from build123d import *

# Parameters (mm, degrees)
F0_R     = 3
F1_DEPTH = 18
F2_R     = 2.1
F3_DEPTH = 10
F4_R     = 1.4
F5_DEPTH = 18.001
F6_SIZE  = 0.5
F7_SIZE  = 0.5


with BuildPart() as f1:
    # F0 (on Front) → F1 (new body)
    with BuildSketch(Plane.XZ):
        Circle(F0_R)
    extrude(amount=-F1_DEPTH)

    # F2 (on face) → F3 (cut)
    with BuildSketch(Plane.XZ):
        Circle(F2_R)
    extrude(amount=-F3_DEPTH, mode=Mode.SUBTRACT)

    # F4 (on Front) → F5 (cut, through all)
    with BuildSketch(Plane.XZ):
        Circle(F4_R)
    extrude(amount=-F5_DEPTH, mode=Mode.SUBTRACT)

    # F6
    f6_edges = [f1.edges().sort_by_distance(p)[0] for p in [
        (-3, 0, 0),
    ]]
    chamfer(f6_edges, length=F6_SIZE)

    # F7
    f7_edges = [f1.edges().sort_by_distance(p)[0] for p in [
        (-3, 18, 0),
    ]]
    chamfer(f7_edges, length=F7_SIZE)


solid = f1.part
Check sheet for the modelled part. Datum: model origin and axes. Units: mm. Give positions to 0.01 mm unless a question says otherwise; leave off trailing zeros. Loops run counter-clockwise (first coordinate to the right, second up) from the corner with the lowest first, then second, coordinate; pieces in that order, holes last. Notation, with made-up numbers: M -37,72.5 L 15,72.5 A15 ccw 15,97.5 Z; hole C 21.25,35 d10. An arc over 180 degrees is marked long. Use a Markdown table: item, result. Add a question column.
Q1. Sectioned sample at D-D, the plane y = 13.25. Record the cut outline in (x, z), then the cut area to 3 significant figures.
Q2. Scan lines: line 1 along Z through (x, y) = (0, 7.5); line 2 along Z through (x, y) = (0, 14.75); line 3 along Y through (x, z) = (1.65, 0.7). Record each from-to range of solid material in increasing order. Write a range as [from, to].
Q3. Sectioned sample at B-B, the plane x = 0. Record the cut outline in (y, z).
Q4. Go/stop test with flat-tipped pins: pin 1 (3 mm diameter, centred on y = 8, z = -2, fed in from -X); pin 2 (1.7 mm diameter, centred on x = 0, z = 0, fed in from -Y). Record where each tip stops, or that it passes through.
Q5. Sectioned sample at C-C, the plane y = 7.75. Record the cut outline in (x, z), then the cut area to 3 significant figures.
Q6. Sectioned sample at A-A, the plane z = 0. Record the cut outline in (x, y).
Q7. Mould release check, pull along X, two halves, no side actions. Record for faces 1 (the cylindrical face through (-3, 9, 0)), 2 (the cylindrical face through (-1.4, 13.94, 0.06)), 3 (the flat face through (1.1, 18, -1.1)): pulls with the +X half, pulls with the -X half, needs draft (parallel to the pull), parting line crosses it, or undercut.
Verdict:
| question | item | result |
|---|---|---|
| 1 | outline | C 0,0 d6; hole C 0,0 d2.8 |
| 1 | area | 22.1 mm^2 |
| 2 | line 1 | [-3, -2.1], [2.1, 3] |
| 2 | line 2 | [-3, -1.4], [1.4, 3] |
| 2 | line 3 | [10, 18] |
| 3 | outline | M 0,-2.5 L 0.5,-3 L 17.5,-3 L 18,-2.5 L 18,-1.4 L 10,-1.4 L 10,-2.1 L 0,-2.1 Z; M 0,2.1 L 10,2.1 L 10,1.4 L 18,1.4 L 18,2.5 L 17.5,3 L 0.5,3 L 0,2.5 Z |
| 4 | pin 1 | x = -2.96 |
| 4 | pin 2 | through |
| 5 | outline | C 0,0 d6; hole C 0,0 d4.2 |
| 5 | area | 14.4 mm^2 |
| 6 | outline | M -3,0.5 L -2.5,0 L -2.1,0 L -2.1,10 L -1.4,10 L -1.4,18 L -2.5,18 L -3,17.5 Z; M 1.4,10 L 2.1,10 L 2.1,0 L 2.5,0 L 3,0.5 L 3,17.5 L 2.5,18 L 1.4,18 Z |
| 7 | face 1 | parting line crosses it |
| 7 | face 2 | undercut |
| 7 | face 3 | needs draft |
